Part model, mm, in its own coordinate system. Face numbers are marked on the shaded views. A direction names the side the tool comes from. Give positions to 0.01 mm unless a question says otherwise; leave off trailing zeros. Order: outer loops, then holes, each group sorted by start corner. A loop starts at its lowest first (then second) coordinate and runs counter-clockwise, first axis right, second up. Notation, with made-up numbers: (85, 10.5) - (117, 10.5) arc R13 ccw to (117, 27.5) - close; hole circle Ø4 at (-13.5, 31). An arc over 180 degrees is marked (long way). One line per item, written item: value.
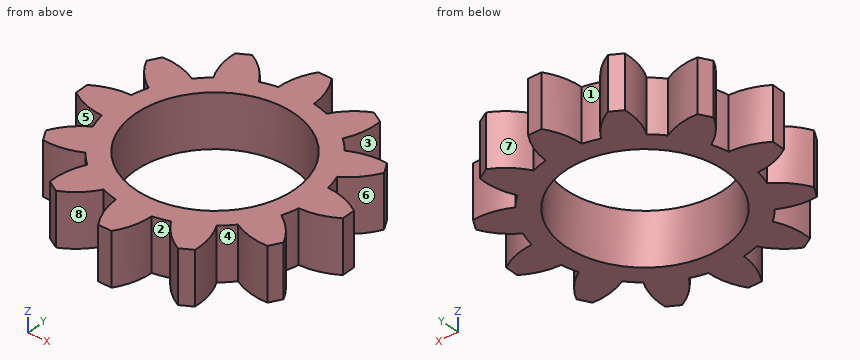
```python
from build123d import *

# Parameters (mm, degrees)
SKETCH1_R           = 12
BOSS_EXTRUDE1_DEPTH = 8


with BuildPart() as part:
    # Sketch1 → Boss-Extrude1 (new body)
    with BuildSketch(Plane(origin=(0, 0, 0), x_dir=(0, 1, 0), z_dir=(0, 0, 1))):
        with BuildLine():
            Line((20, 1), (20, -1))
            ThreePointArc((20, -1), (17.497232023, -2.204975942), (14.759551992, -2.675))
            ThreePointArc((14.759551992, -2.675), (14.488887394, -3.882285677), (14.119646973, -5.063158041))
            ThreePointArc((14.119646973, -5.063158041), (16.262701001, -6.832536438), (17.820508076, -9.133974596))
            Line((17.820508076, -9.133974596), (16.820508076, -10.866025404))
            ThreePointArc((16.820508076, -10.866025404), (14.050559457, -10.658181192), (11.444646973, -9.696393951))
            ThreePointArc((11.444646973, -9.696393951), (10.606601718, -10.606601718), (9.696393951, -11.444646973))
            ThreePointArc((9.696393951, -11.444646973), (10.667643983, -14.048500628), (10.866025404, -16.820508076))
            Line((10.866025404, -16.820508076), (9.133974596, -17.820508076))
            ThreePointArc((9.133974596, -17.820508076), (6.839050831, -16.255535399), (5.063158041, -14.119646973))
            ThreePointArc((5.063158041, -14.119646973), (3.882285677, -14.488887394), (2.675, -14.759551992))
            ThreePointArc((2.675, -14.759551992), (2.214200373, -17.50018042), (1, -20))
            Line((1, -20), (-1, -20))
            ThreePointArc((-1, -20), (-2.204975942, -17.497232023), (-2.675, -14.759551992))
            ThreePointArc((-2.675, -14.759551992), (-3.882285677, -14.488887394), (-5.063158041, -14.119646973))
            ThreePointArc((-5.063158041, -14.119646973), (-6.832536438, -16.262701001), (-9.133974596, -17.820508076))
            Line((-9.133974596, -17.820508076), (-10.866025404, -16.820508076))
            ThreePointArc((-10.866025404, -16.820508076), (-10.658181192, -14.050559457), (-9.696393951, -11.444646973))
            ThreePointArc((-9.696393951, -11.444646973), (-10.606601718, -10.606601718), (-11.444646973, -9.696393951))
            ThreePointArc((-11.444646973, -9.696393951), (-14.048500628, -10.667643983), (-16.820508076, -10.866025404))
            Line((-16.820508076, -10.866025404), (-17.820508076, -9.133974596))
            ThreePointArc((-17.820508076, -9.133974596), (-16.255535399, -6.839050831), (-14.119646973, -5.063158041))
            ThreePointArc((-14.119646973, -5.063158041), (-14.488887394, -3.882285677), (-14.759551992, -2.675))
            ThreePointArc((-14.759551992, -2.675), (-17.50018042, -2.214200373), (-20, -1))
            Line((-20, -1), (-20, 1))
            ThreePointArc((-20, 1), (-17.497232023, 2.204975942), (-14.759551992, 2.675))
            ThreePointArc((-14.759551992, 2.675), (-14.488887394, 3.882285677), (-14.119646973, 5.063158041))
            ThreePointArc((-14.119646973, 5.063158041), (-16.262701001, 6.832536438), (-17.820508076, 9.133974596))
            Line((-17.820508076, 9.133974596), (-16.820508076, 10.866025404))
            ThreePointArc((-16.820508076, 10.866025404), (-14.050559457, 10.658181192), (-11.444646973, 9.696393951))
            ThreePointArc((-11.444646973, 9.696393951), (-10.606601718, 10.606601718), (-9.696393951, 11.444646973))
            ThreePointArc((-9.696393951, 11.444646973), (-10.667643983, 14.048500628), (-10.866025404, 16.820508076))
            Line((-10.866025404, 16.820508076), (-9.133974596, 17.820508076))
            ThreePointArc((-9.133974596, 17.820508076), (-6.839050831, 16.255535399), (-5.063158041, 14.119646973))
            ThreePointArc((-5.063158041, 14.119646973), (-3.882285677, 14.488887394), (-2.675, 14.759551992))
            ThreePointArc((-2.675, 14.759551992), (-2.214200373, 17.50018042), (-1, 20))
            Line((-1, 20), (1, 20))
            ThreePointArc((1, 20), (2.204975942, 17.497232023), (2.675, 14.759551992))
            ThreePointArc((2.675, 14.759551992), (3.882285677, 14.488887394), (5.063158041, 14.119646973))
            ThreePointArc((5.063158041, 14.119646973), (6.832536438, 16.262701001), (9.133974596, 17.820508076))
            Line((9.133974596, 17.820508076), (10.866025404, 16.820508076))
            ThreePointArc((10.866025404, 16.820508076), (10.658181192, 14.050559457), (9.696393951, 11.444646973))
            ThreePointArc((9.696393951, 11.444646973), (10.606601718, 10.606601718), (11.444646973, 9.696393951))
            ThreePointArc((11.444646973, 9.696393951), (14.048500628, 10.667643983), (16.820508076, 10.866025404))
            Line((16.820508076, 10.866025404), (17.820508076, 9.133974596))
            ThreePointArc((17.820508076, 9.133974596), (16.255535399, 6.839050831), (14.119646973, 5.063158041))
            ThreePointArc((14.119646973, 5.063158041), (14.488887394, 3.882285677), (14.759551992, 2.675))
            ThreePointArc((14.759551992, 2.675), (17.50018042, 2.214200373), (20, 1))
        make_face()
        with Locations(Location((0, 0, 0), (0, 0, 270))):
            Circle(SKETCH1_R, mode=Mode.SUBTRACT)
    extrude(amount=BOSS_EXTRUDE1_DEPTH)


solid = part.part
```
1) Cut at D-D, the plane x = -13.5. Give the cut face in (y, z), then the cut area to 3 significant figures.
Outcome:
outline: (-10.53, 0) - (10.52, 0) - (10.52, 8) - (-10.53, 8) - close
area: 168 mm^2
2) Mould opens along Y. For the marked faces 1, 2 and 3 say: released by +Y, released by -Y, zero draft, split by the parting line, or undercut.
Outcome:
face 1: released by +Y
face 2: released by -Y
face 3: undercut
3) Drill centre lines: line 1 along X through (y, z) = (-10, 4); line 2 along Y through (x, z) = (-15, 7.75); line 3 along Y through (x, z) = (0, 2.25). Where is each one in solid material? Low to high. Write a range as from..to.
Outcome:
line 1: x = -17.32..-12.05, -11.18..-6.63, 6.63..11.18, 12.06..17.32
line 2: y = -10.83..-5.68, -2.67..2.66, 5.67..10.82
line 3: y = -20..-12, 12..20
4) Cut at A-A, the plane y = 0. Give the cut face in (x, z).
Outcome:
outline: (-20, 0) - (-12, 0) - (-12, 8) - (-20, 8) - close; (12, 0) - (20, 0) - (20, 8) - (12, 8) - close
5) Pin check, flat tips, straight feed: pin 1 (4 mm diameter, centred on x = -12, z = 3.5, fed in from -Y); pin 2 (3 mm diameter, centred on x = 5, z = 4.5, fed in from +Y); pin 3 (3 mm diameter, centred on x = -7, z = 6.5, fed in from -Y). Stop position of each tip, or through.
Outcome:
pin 1: stops at y = -17.32
pin 2: stops at y = 15.95
pin 3: stops at y = -17.48
6) Which spindle directions (+Z, -Z, +X, -X, +Y, -Y) get a long thin tool onto all of the face, cutting with end or side? Do the marked faces 4, 5, 6, 7 and 8. Say none if no direction does.
Outcome:
face 4: +Z, -Z
face 5: +Z, -Z, -X
face 6: +Z, -Z, +X
face 7: +Z, -Z, +Y
face 8: +Z, -Z, -Y
7) Cut at C-C, the plane y = 15.5. Give the cut face in (x, z), then the cut area to 3 significant figures.
Outcome:
outline: (-10.87, 0) - (-6.09, 0) - (-6.09, 8) - (-10.87, 8) - close; (-2.63, 0) - (2.62, 0) - (2.62, 8) - (-2.63, 8) - close; (6.08, 0) - (10.86, 0) - (10.86, 8) - (6.08, 8) - close
area: 119 mm^2
